Design review of the part shown in the three views and the two pictorial views. Dimensions are in mm from the part's minimum x, y and z. A direction names the side the tool comes from. Round coordinates to 2 decimals unless told otherwise and drop trailing zeros. Order: outer loops, then holes, each group sorted by start corner. A loop starts at its lowest first (then second) coordinate and runs counter-clockwise, first axis right, second up.
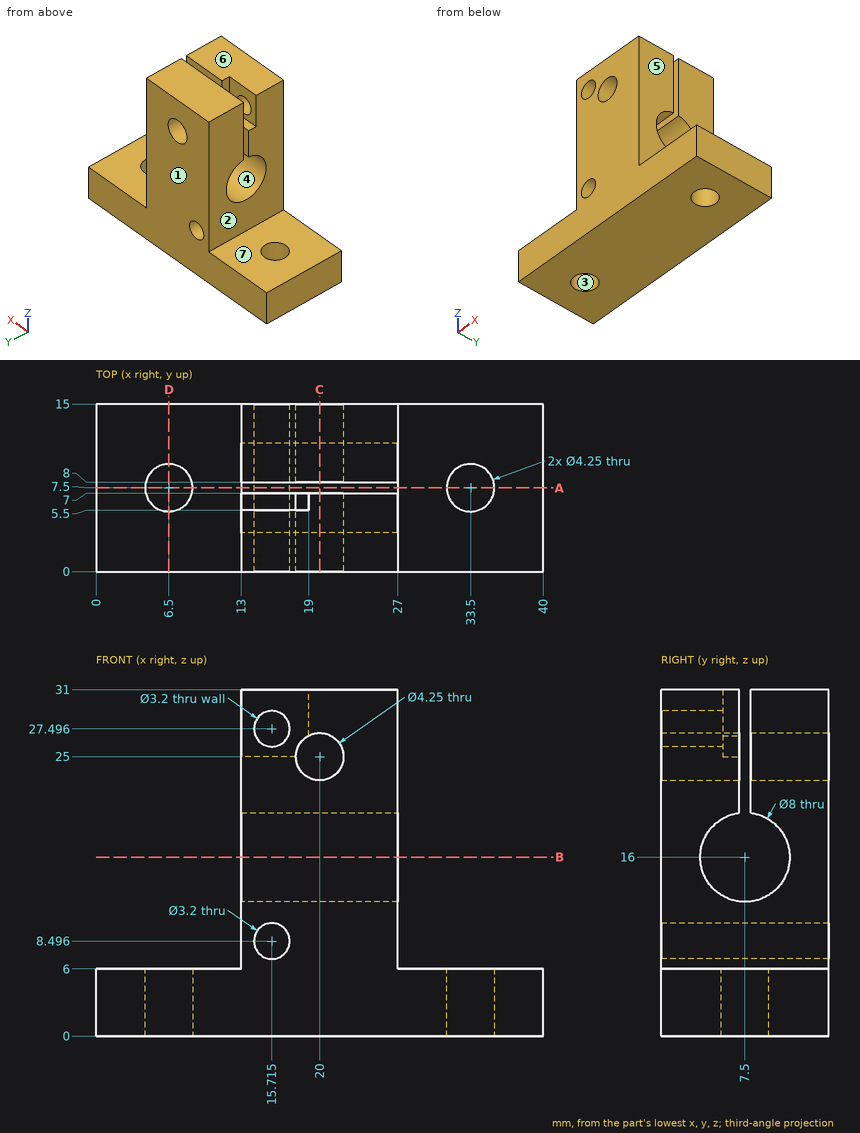
(1) Add section A-A on y = 7.5. Give the boundary of the cut face in (x, z) (1 decimal), plus the area to 3 significant figures.
(2) Tool access review of the marked faces 5, 6 and 7: name each direction out of +Z, -Z, +X, -X, +Y, -Y from which nothing blocks a thin tool from reaching the whole face with its end or side.
(3) Wall thickness on L1, parallel to Y at x = 6.5, z = 2.3 (1 decimal); L2, parallel to Y at x = 21.5, z = 27.5; L3, parallel to X at y = 3, z = 20: over which ranges is each line inside the solid? List them lowest first.
(4) Add section C-C on x = 20. Give the boundary of the cut face in (y, z) (1 decimal), plus the area to 3 significant figures.
(5) Draft analysis for pull direction Y (two halves, no side actions). For the marked faces 1, 2, 3 and 4, state which applies: pulls with the +Y half, pulls with the -Y half, needs draft (parallel to the pull), parting line crosses it, or undercut.
(6) Clearance check with flat-ended pins moving along their axes: P1, Ø1.5, axis at x = 16, z = 19, coming from the -Y side; P2, Ø4, axis at x = 20, z = 25, coming from the -Y side; P3, Ø1.2, axis at y = 6.5, z = 29.5, coming from the -X side; P4, Ø6, axis at y = 11.5, z = 24.5, coming from the +X side. State where each tip first meets the part, or that it passes through.
(7) Add section D-D on x = 6.5. Give the boundary of the cut face in (y, z) (1 decimal), plus the area to 3 significant figures.
(8) Add section B-B on z = 16. Give the boundary of the cut face in (x, y).
Here are the results:
1. outline: (0, 0) - (4.4, 0) - (4.4, 6) - (0, 6) - close; (8.6, 0) - (31.4, 0) - (31.4, 6) - (27, 6) - (27, 12) - (13, 12) - (13, 6) - (8.6, 6) - close; (35.6, 0) - (40, 0) - (40, 6) - (35.6, 6) - close; hole circle Ø3.2 at (15.7, 8.5)
1. area: 265 mm2
2. face 5: +Z, +X, +Y, -Y
2. face 6: +Z, +X, -X, +Y, -Y
2. face 7: +Z, -X, +Y, -Y
3. L1: y = 0 to 5.4, 9.6 to 15
3. L2: y = 0 to 7, 8 to 15
3. L3: x = 13 to 27
4. outline: (0, 0) - (15, 0) - (15, 22.9) - (8, 22.9) - (8, 20) arc R4 cw (long way) to (7, 20) - (7, 22.9) - (0, 22.9) - close; (0, 27.1) - (7, 27.1) - (7, 31) - (0, 31) - close; (8, 27.1) - (15, 27.1) - (15, 31) - (8, 31) - close
4. area: 344 mm2
5. face 1: pulls with the +Y half
5. face 2: needs draft
5. face 3: undercut
5. face 4: undercut
6. P1: stops at y = 0
6. P2: passes through
6. P3: stops at x = 19
6. P4: stops at x = 27
7. outline: (0, 0) - (5.4, 0) - (5.4, 6) - (0, 6) - close; (9.6, 0) - (15, 0) - (15, 6) - (9.6, 6) - close
7. area: 64.5 mm2
8. outline: (13, 0) - (27, 0) - (27, 3.5) - (13, 3.5) - close; (13, 11.5) - (27, 11.5) - (27, 15) - (13, 15) - close
